The model under review builds one solid part; all positions refer to its coordinate system, in mm. A direction names the side the tool comes from. Round coordinates to 2 decimals unless told otherwise and drop trailing zeros. Write each loop counter-clockwise with the first axis right and the second up, starting at its lowest first coordinate (ties: lowest second). Pieces come first, ordered by that corner, then holes. Notation, with made-up numbers: M -21,60.5 L 5,60.5 A18 ccw 5,95.5 Z; hole C -16.75,-5 d3. An arc over 180 degrees is marked long. Write item = value, one per line. Start each with the question number.
Item 1: For pin 1 Ø8 at (y, z) = (35, 29) entering from -X; pin 2 Ø4 at (x, z) = (34.25, 5) entering from -Y; pin 3 Ø3 at (y, z) = (6.5, 3.5) entering from +X; pin 4 Ø1 at (y, z) = (12, -16.5) entering from +X, all flat-tipped, find the tip position at first contact; note any pin that passes through.
Item 2: Tool access review of faces 4 (the cylindrical face through (-39.96, 30.68, -1.76)), 5 (the flat face through (-22, 50, -34)): name each direction out of +Z, -Z, +X, -X, +Y, -Y from which nothing blocks a thin tool from reaching the whole face with its end or side.
Item 3: Take a section at A-A, the plane x = 0. Give the boundary of the cut face in (y, z) (3 decimals).
Item 4: Take a section at C-C, the plane y = 9. Give the boundary of the cut face in (x, z), plus the area to 3 significant figures.
Item 5: Take a section at D-D, the plane y = 47.5. Give the boundary of the cut face in (x, z).
Item 6: To check wall thickness, follow line 1 along Z through (x, y) = (34.25, 7.25); line 2 along Z through (x, y) = (-15, 5); line 3 along X through (y, z) = (5.5, 5). State the ranges of each line that lie inside material, in increasing order.
Item 7: Take a section at B-B, the plane z = 0. Give the boundary of the cut face in (x, y) (3 decimals).
Item 8: The part is to be moulded in two halves that separate along X. For faces 1 (the cylindrical face through (-18.5, 6, 4.9)), 2 (the cylindrical face through (47.69, 35.21, -15.02)), 3 (the flat face through (7, 0, 0)), say which applies: +X half, -X half, draft (parallel to the pull), parting line (faces both ways), or undercut.
from build123d import *

# Parameters (mm, degrees)
FILLET1_R          = 20
SKETCH6_W          = 39.5
SKETCH6_H          = 20
SKETCH6_R          = 6.375
CUT_EXTRUDE1_DEPTH = 9.9
SKETCH8_R          = 6.375
CUT_EXTRUDE2_DEPTH = 37.9
SKETCH9_R          = 3.25
CUT_EXTRUDE3_DEPTH = 37.9


with BuildPart() as part:
    # Sketch5 → Revolve1 (revolve)
    with BuildSketch(Plane.XY, mode=Mode.PRIVATE) as revolve1_sk:
        Polygon((0, 0), (-50, 0), (-50, 50), (-40, 50), (-40, 11.9), (0, 11.9), align=None)
    revolve(revolve1_sk.sketch.rotate(Axis((0, 0, 0), (0, 1, 0)), 180), axis=Axis((0, 0, 0), (0, 1, 0)))

    # Fillet1
    fillet1_edges = [part.edges().sort_by_distance(p)[0] for p in [
        (-50, 0, 0),
    ]]
    fillet(fillet1_edges, radius=FILLET1_R)

    # Sketch6 → Cut-Extrude1 (cut)
    with BuildSketch(Plane(origin=(0, 11.9, 0), x_dir=(1, 0, 0), z_dir=(0, 1, 0))):
        with Locations((9.5, 0)):
            Rectangle(SKETCH6_W, SKETCH6_H)
        with Locations(Location((0, 0, 0), (0, 0, 180))):
            Circle(SKETCH6_R, mode=Mode.SUBTRACT)
    extrude(amount=-CUT_EXTRUDE1_DEPTH, mode=Mode.SUBTRACT)

    # Sketch8 → Cut-Extrude2 (cut)
    with BuildSketch(Plane(origin=(0, 11.9, 0), x_dir=(1, 0, 0), z_dir=(0, 1, 0))):
        with Locations(Location((0, 0, 0), (0, 0, 270))):
            Circle(SKETCH8_R)
    extrude(amount=-CUT_EXTRUDE2_DEPTH, mode=Mode.SUBTRACT)

    # Sketch9 → Cut-Extrude3 (cut)
    with BuildSketch(Plane(origin=(0, 11.9, 0), x_dir=(1, 0, 0), z_dir=(0, 1, 0))):
        with Locations(Location((-15.25, 5, 0), (0, 0, 180))):
            Circle(SKETCH9_R)
        with Locations(Location((34.25, 5, 0), (0, 0, 131.634247299))):
            Circle(SKETCH9_R)
        with Locations(Location((34.25, -5, 0), (0, 0, 180))):
            Circle(SKETCH9_R)
        with Locations((-15.25, -5)):
            Circle(SKETCH9_R)
    extrude(amount=-CUT_EXTRUDE3_DEPTH, mode=Mode.SUBTRACT)


solid = part.part
Response values:
q1.pin_1 = -43.3
q1.pin_2 = through
q1.pin_3 = 45.87
q1.pin_4 = 45.71
q2.face_4 = +Y
q2.face_5 = +Z, -Z, +X, -X, +Y
q3.outline = M 0,-30 A20 ccw 20,-50 L 50,-50 L 50,-40 L 11.9,-40 L 11.9,-10 L 2,-10 L 2,-6.375 L 0,-6.375 Z; M 0,6.375 L 2,6.375 L 2,10 L 11.9,10 L 11.9,40 L 50,40 L 50,50 L 20,50 A20 ccw 0,30 Z
q4.outline = C 0,0 d93.41; hole C -15.25,-5 d6.5; hole C -15.25,5 d6.5; hole M -10.25,-10 L 29.25,-10 L 29.25,10 L -10.25,10 Z; hole C 34.25,-5 d6.5; hole C 34.25,5 d6.5
q4.area = 5,930 mm2
q5.outline = C 0,0 d100; hole C 0,0 d80
q6.line_1 = -29.81 to -8.25, -1.75 to 1.75, 8.25 to 29.81
q6.line_2 = -40.54 to -8.24, -1.76 to 1.76, 8.24 to 40.54
q6.line_3 = -43.49 to -18.5, -12 to -10.25, 29.25 to 31, 37.5 to 43.49
q7.outline = M -50,20 A20 ccw -30,0 L -6.375,0 L -6.375,2 L -10.25,2 L -10.25,11.9 L -40,11.9 L -40,50 L -50,50 Z; M 6.375,0 L 30,0 A20 ccw 50,20 L 50,50 L 40,50 L 40,11.9 L 29.25,11.9 L 29.25,2 L 6.375,2 Z
q8.face_1 = undercut
q8.face_2 = parting line
q8.face_3 = draft
